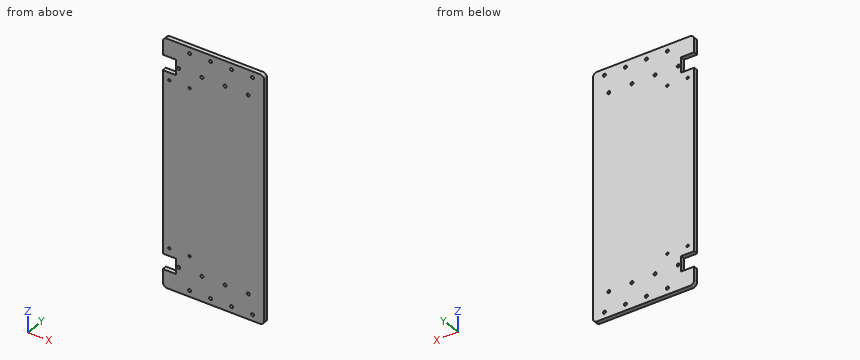
Autodesk Inventor part; units mm, degrees
ref_plane "Arbeitsebene1" through (0, 0, 0) normal (0, 0, 1) x (1, 0, 0)
ref_plane "YZ Plane" through (0, 0, 0) normal (1, 0, 0) x (0, 1, 0)
ref_plane "XZ Plane" through (0, 0, 0) normal (0, 1, 0) x (-1, 0, 0)
sketch "Skizze1" plane through (0, 0, 0) normal (0, 1, 0) x (-1, 0, 0)
  line L0 (-70, 170) -> (70, 170)
  line L1 (70, 170) -> (70, -170)
  line L2 (70, -170) -> (-70, -170)
  line L3 (-70, -170) -> (-70, 170)
  line L4 (-70, 170) -> (70, -170) construction
  line L5 (70, 170) -> (-70, -170) construction
  point P0 (0, 0)
  dimension "d0" = 340
  dimension "d1" = 140
extrude "Extrusion1" add sketch "Skizze1" along normal blind 6
sketch "Skizze2" plane through (0, 6, 0) normal (0, 1, 0) x (1, 0, 0)
  line L0 (-70, 170) -> (-70, -170)
  line L1 (-70, -146) -> (-52, -146)
  line L2 (-52, -146) -> (-52, -125)
  line L3 (-52, -125) -> (-70, -125)
  line L4 (-70, 125) -> (-52, 125)
  line L5 (-52, 125) -> (-52, 146)
  line L6 (-52, 146) -> (-70, 146)
  line L7 (-70, -170) -> (70, -170)
  line L8 (70, 170) -> (-70, 170)
  point P0 (0, 0)
  dimension "d4" = 21
  dimension "d5" = 21
  dimension "d6" = 24
  dimension "d7" = 24
  dimension "d8" = 18
extrude "Extrusion2" cut sketch "Skizze2" against normal up to surface (6 mm away)
sketch "Skizze3" plane through (0, 6, 0) normal (0, 1, 0) x (1, 0, 0)
  line L0 (70, -170) -> (70, 170)
  line L1 (-52, -125) -> (-52, -146)
  point P0 (0, 0)
  point P1 (-48, -135.5)
  point P2 (-16, -135.5)
  point P3 (16, -135.5)
  point P4 (48, -135.5)
  point P5 (-52, -135.5)
  dimension "d11" = 22
  dimension "d12" = 32
  dimension "d13" = 32
  dimension "d14" = 32
hole "Bohrung1" at (-48, 6, 135.5) at (-16, 6, 135.5) at (16, 6, 135.5) at (48, 6, 135.5) direction (0, -1, 0) diameter 4.134 depth 6
fillet "Rundung1" radius 6 4 edges at (-70, 3, 170) (70, 3, 170) (70, 3, -170) (-70, 3, -170)
sketch "Skizze4" plane through (0, 6, 0) normal (0, 1, 0) x (1, 0, 0)
  circle A0 centre (48, -135.5) radius 2.067
  line L0 (70, -164) -> (70, 164)
  point P0 (0, 0)
  point P1 (54, -161.5)
  point P2 (25, -161.5)
  point P3 (-4, -161.5)
  point P4 (-33, -161.5)
  dimension "d23" = 26
  dimension "d24" = 16
  dimension "d25" = 29
  dimension "d26" = 29
  dimension "d27" = 29
hole "Bohrung2" at (54, 6, 161.5) at (25, 6, 161.5) at (-4, 6, 161.5) at (-33, 6, 161.5) direction (0, -1, 0) diameter 4.134 depth 6
ref_plane "Arbeitsebene1" through (0, 0, 0) normal (0, 0, 1) x (1, 0, 0)
mirror "Spiegeln1" about plane through (0, 0, 0) normal (0, 0, 1) of "Bohrung2", "Bohrung1"
sketch "Skizze5" plane through (0, 6, 0) normal (0, 1, 0) x (1, 0, 0)
  line L0 (-70, -125) -> (-52, -125)
  point P0 (0, 0)
  point P1 (-61, -114.5)
  point P2 (-61, 114.5)
  point P3 (-61, -125)
  dimension "d36" = 114.5
  dimension "d37" = 114.5
hole "Bohrung3" at (-61, 6, 114.5) at (-61, 6, -114.5) direction (0, -1, 0) diameter 3.242 depth 6
sketch "Skizze6" plane through (0, 6, 0) normal (0, 1, 0) x (1, 0, 0)
  line L0 (-52, -125) -> (-52, -146)
  point P0 (0, 0)
  point P1 (-33, -114.5)
  point P2 (-33, 114.5)
  dimension "d45" = 19
  dimension "d46" = 114.5
  dimension "d47" = 114.5
hole "Bohrung4" at (-33, 6, 114.5) at (-33, 6, -114.5) direction (0, -1, 0) diameter 3.242 depth 6
properties part number "1011"
The listing builds one solid part. Answer for the finished solid, in the listing's coordinates (mm). Round coordinates to 2 decimals unless told otherwise and drop trailing zeros. Write each question's results on one line, items separated by ' | '. Start each with the question number.
Item 1: Straight lines are drawn through the part: L1, parallel to X at y = 4, z = 135.5; L2, parallel to Z at x = -57.5, y = 3.5; L3, parallel to Z at x = 16, y = 3.95. For each, find the intervals that lie inside material, in ascending order. Write a range as [from, to].
Item 2: A flat-ended cylindrical pin translates along its axis: pin 1 Ø1.8 at (y, z) = (2.5, -137) entering from -X. Find the tip coordinate at first contact, or state that the pin passes through.
Item 3: A cutting plane is placed at A-A on y = 4.8. State how many separate pieces and enclosed holes the cut face has, and give its area (3 significant figures).
Check sheet entries:
1) L1: [-52, -50.07], [-45.93, -18.07], [-13.93, 13.93], [18.07, 45.93], [50.07, 70] | L2: [-170, -146], [-125, 125], [146, 170] | L3: [-170, -137.57], [-133.43, 133.43], [137.57, 170]
2) pin 1: x = -52
3) separate pieces: 1 | enclosed holes: 20 | area: 46,600 mm²
